Autodesk Fusion 360 part; units mm, degrees
sketch "Boceto1" plane through (0, 0, 0) normal (1, 0, 0) x (0, 1, 0)
  line L0 (0, 0) -> (-0.8775, 0)
  line L1 (0, 5) -> (-0.8775, 5)
  line L2 (130, 0) -> (130.8775, 0)
  line L3 (130, 5) -> (130.8775, 5)
  arc A0 (-0.8775, 5) -> (-0.8775, 0) centre (-4, 2.5) ccw
  line L4 (78.1225, 0) -> (130, 0)
  line L5 (130, 5) -> (78.1225, 5)
  line L6 (75.0004, 5) -> (74.9996, 5)
  arc A1 (78.1225, 5) -> (71.8775, 5) centre (75, 2.5) ccw
  arc A2 (71.8775, 0) -> (78.1225, 0) centre (75, 2.5) ccw
  arc A3 (130.8775, 0) -> (130.8775, 5) centre (134, 2.5) ccw
  line L7 (0, 0) -> (61.8775, 0)
  line L8 (71.8775, 5) -> (68.1225, 5)
  line L9 (61.8775, 5) -> (0, 5)
  arc A4 (61.8775, 0) -> (68.1225, 0) centre (65, 2.5) ccw
  arc A5 (68.1225, 5) -> (61.8775, 5) centre (65, 2.5) ccw
  line L10 (0, 0) -> (65, 0)
  line L11 (68.1225, 0) -> (71.8775, 0)
  line L12 (0, 0) -> (61.8775, 0)
  line L13 (68.1225, 0) -> (71.8775, 0)
  circle A6 centre (-4, 2.5) radius 1.5
  circle A7 centre (65, 2.5) radius 1.5
  circle A8 centre (75, 2.5) radius 1.5
  circle A9 centre (134, 2.5) radius 1.5
  dimension "d1" = 130
  dimension "d2" = 5
  dimension "d7" = 8
  dimension "d9" = 65
  dimension "d10" = 2.5
  dimension "d11" = 8
  dimension "d15" = 3
  dimension "d16" = 3
  dimension "d17" = 3
  dimension "d18" = 3
extrude "Extruir2" add sketch "Boceto1" along normal blind 1.5
Can you work these out from the model? Positions are in its coordinate system, mm. Round coordinates to 2 decimals unless told otherwise and drop trailing zeros. Write each loop counter-clockwise with the first axis right and the second up, starting at its lowest first coordinate (ties: lowest second). Pieces come first, ordered by that corner, then holes. Notation, with made-up numbers: (56, -2) - (86, -2) arc R30 cw to (86, 20) - close; hole circle Ø10 at (84, 37). An arc over 180 degrees is marked (long way). Write each question's results on one line, items separated by ' | '. Start each with the question number.
1) Suppose I cut it at B-B (z = 2.5). List the corners of the cut face in (x, y) for me, and give its area (3 significant figures).
2) Please list where these lines run through material, in increasing order: line 1 (Y direction, x = 0.65, z = 2.25); line 2 (Z direction, x = 0.45, y = 134); line 3 (Y direction, x = 1.1, z = -0.5).
3) We'd pull the mould along Y, two halves only. Please class faces 1 (the cylindrical face through (0.7, -8, 2.4)), 2 (the flat face through (0, 64, 4)), 3 (the cylindrical face through (0.74, 132.5, 2.43)): released by +Y, released by -Y, zero draft, split by the parting line, or undercut.
4) Suppose I cut it at D-D (y = 91). List the corners of the cut face in (x, z) for me, and give its area (3 significant figures).
5) Suppose I cut it at A-A (x = 0.5). List the corners of the cut face in (y, z) for me.
6) Suppose I cut it at C-C (y = -4). List the corners of the cut face in (x, z) for me.
7) For pin 1 Ø4 at (y, z) = (48, 3) entering from -X, with a flat end and sliding along its axis, tell me the tip position at first contact or that it passes through.
Here are the results:
1) outline: (0, -8) - (1.5, -8) - (1.5, -5.5) - (0, -5.5) - close; (0, -2.5) - (1.5, -2.5) - (1.5, 63.5) - (0, 63.5) - close; (0, 66.5) - (1.5, 66.5) - (1.5, 73.5) - (0, 73.5) - close; (0, 76.5) - (1.5, 76.5) - (1.5, 132.5) - (0, 132.5) - close; (0, 135.5) - (1.5, 135.5) - (1.5, 138) - (0, 138) - close | area: 201 mm2
2) line 1: y = -7.99 to -5.48, -2.52 to 63.52, 66.48 to 73.52, 76.48 to 132.52, 135.48 to 137.99 | line 2: z = -1.5 to 1, 4 to 6.5 | line 3: y = -6.65 to -1.35, 62.35 to 67.65, 72.35 to 77.65, 131.35 to 136.65
3) face 1: undercut | face 2: zero draft | face 3: undercut
4) outline: (0, 0) - (1.5, 0) - (1.5, 5) - (0, 5) - close | area: 7.50 mm2
5) outline: (-0.88, 0) - (61.88, 0) arc R4 ccw to (68.12, 0) - (71.88, 0) arc R4 ccw to (78.12, 0) - (130.88, 0) arc R4 ccw (long way) to (130.88, 5) - (78.12, 5) arc R4 ccw to (71.88, 5) - (68.12, 5) arc R4 ccw to (61.88, 5) - (-0.88, 5) arc R4 ccw (long way) to start; hole circle Ø3 at (-4, 2.5); hole circle Ø3 at (65, 2.5); hole circle Ø3 at (75, 2.5); hole circle Ø3 at (134, 2.5)
6) outline: (0, -1.5) - (1.5, -1.5) - (1.5, 1) - (0, 1) - close; (0, 4) - (1.5, 4) - (1.5, 6.5) - (0, 6.5) - close
7) pin 1: stops at x = 0
